Source: CAD feature listing. Evaluate the final solid. Frame: model axes, mm. A direction names the side the tool comes from. Coordinates: 2 decimals unless noted, no trailing zeros. Loops run counter-clockwise (first coordinate to the right, second up) from the corner with the lowest first, then second, coordinate; pieces in that order, holes last. Notation, with made-up numbers: (84, 80) -> (125, 80) arc R23 ccw to (125, 117) -> close; hole circle Ø10 at (49, 26). An arc over 180 degrees is marked (long way). Answer as CSV lines item,"result".
Autodesk Fusion 360 part; units mm, degrees
sketch "Sketch1" plane through (0, 0, 0) normal (0, 0, 1) x (1, 0, 0)
  line L0 (0, 50) -> (23, 50)
  line L1 (23, 50) -> (23, 23)
  line L2 (23, 23) -> (0, 23)
  line L3 (0, 23) -> (0, 50)
  line L4 (0, 23) -> (1, 23)
  line L5 (1, 23) -> (1, 50)
  line L6 (1, 50) -> (0, 50)
  line L7 (0, 50) -> (0, 23)
  dimension "d1" = 23
  dimension "d2" = 27
extrude "Extrude1" add sketch "Sketch1" along normal blind 1 contours L0 L1 L2 L5
extrude "Extrude2" add sketch "Sketch1" along normal blind 2.5 contours L0 L2 L3 L4 L5 L6 L7
(1) Cut plane A-A (x = 15.5). Return the cut outline in (y, z).
Computed values:
outline,"(23, 0) -> (50, 0) -> (50, 1) -> (23, 1) -> close"
(2) Cut plane C-C (z = 2). Return the cut outline in (x, y).
Computed values:
outline,"(0, 23) -> (1, 23) -> (1, 50) -> (0, 50) -> close"
(3) Access query for faces 1 (the flat face through (1, 36, 2)), 2 (the flat face through (11.7, 23, 0.4)). Directions: +Z, -Z, +X, -X, +Y, -Y. A direction counts if a zero-diameter tool reaches every point of the face in a straight line with its end or side. Return the directions, or none.
Computed values:
face 1,"+Z, +X, +Y, -Y"
face 2,"+Z, -Z, +X, -X, -Y"
(4) Material intervals for L1, parallel to Z at x = 1.75, y = 36.25, sorted ascending. Write a range as [from, to].
Computed values:
L1,"[0, 1]"
(5) Pin query (flat end, axial travel): pin 1 Ø10 at (x, y) = (6, 45.5) entering from -Z; pin 2 Ø1.2 at (y, z) = (39.5, 2) entering from +X; pin 3 Ø6.5 at (x, y) = (15, 30.5) entering from +Z. Return the tip coordinate at first contact, or that it passes through.
Computed values:
pin 1,"z = 0"
pin 2,"x = 1"
pin 3,"z = 1"
(6) Cut plane B-B (y = 43.5). Return the cut outline in (x, z), then the cut area to 3 significant figures.
Computed values:
outline,"(0, 0) -> (23, 0) -> (23, 1) -> (1, 1) -> (1, 2.5) -> (0, 2.5) -> close"
area,"24.5 mm^2"
